Design review of the part shown in the three views and the two pictorial views. Dimensions are in mm from the part's minimum x, y and z. A direction names the side the tool comes from. Round coordinates to 2 decimals unless told otherwise and drop trailing zeros. Order: outer loops, then holes, each group sorted by start corner. A loop starts at its lowest first (then second) coordinate and runs counter-clockwise, first axis right, second up.
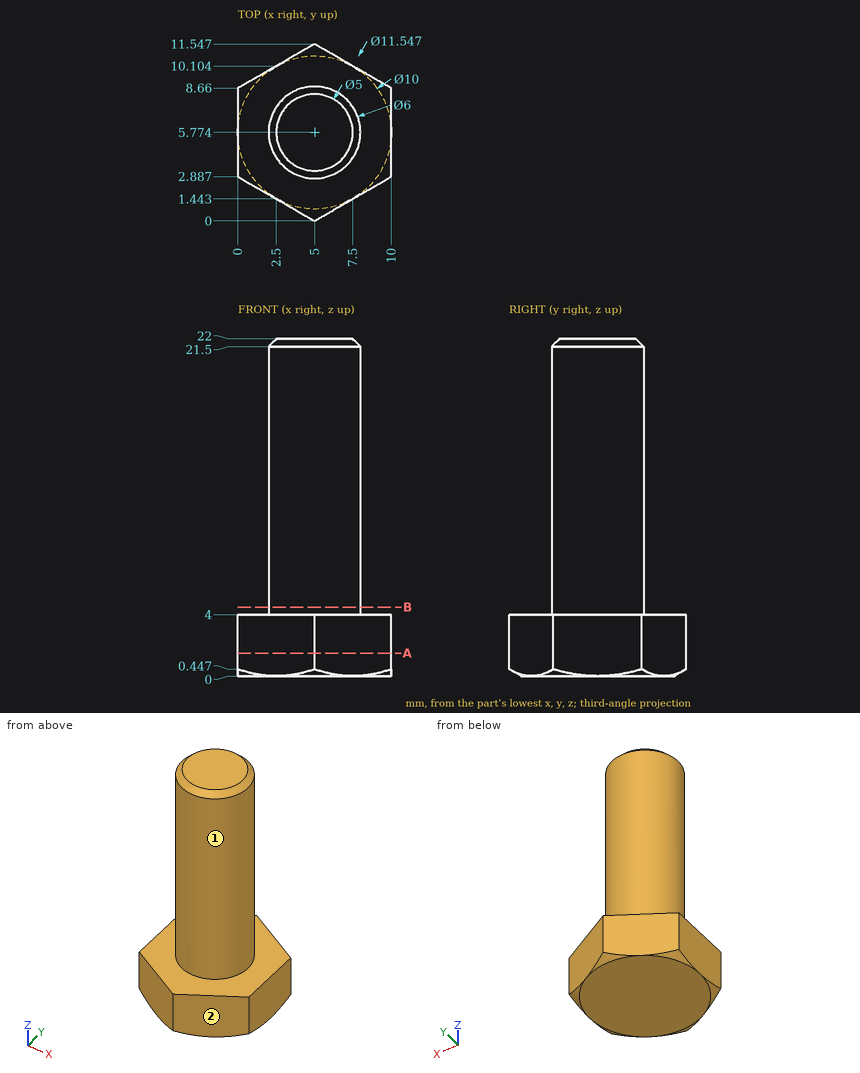
1) Clearance check with flat-ended pins moving along their axes: P1, Ø2, axis at y = 6.5, z = 10, coming from the +X side; P2, Ø1.5, axis at y = 5, z = 11.5, coming from the -X side; P3, Ø1, axis at x = 2, z = 13, coming from the +Y side. State where each tip first meets the part, or that it passes through.
Results:
P1: stops at x = 8
P2: stops at x = 2
P3: stops at y = 7.43
2) Take a section at B-B on z = 4.5. Give the boundary of the cut face in (x, y).
Results:
outline: circle Ø6 at (5, 5.77)
3) For the marked faces 1 and 2, list the 3-axis set-ups (+Z, -Z, +X, -X, +Y, -Y) from which the entire face can be reached by the end or side of a thin tool; tool diameter is ignored.
Results:
face 1: +Z
face 2: +Z, -Z, +X, -Y
4) Take a section at A-A on z = 1.5. Give the boundary of the cut face in (x, y), plus the area to 3 significant figures.
Results:
outline: (0, 2.89) - (5, 0) - (10, 2.89) - (10, 8.66) - (5, 11.55) - (0, 8.66) - close
area: 86.6 mm2
5) To check wall thickness, follow line 1 along X through (y, z) = (5.75, 17.25); line 2 along Z through (x, y) = (0.5, 6.5); line 3 along X through (y, z) = (8, 11.5). State the ranges of each line that lie inside material, in increasing order.
Results:
line 1: x = 2 to 8
line 2: z = 0 to 4
line 3: x = 2.99 to 7.01
